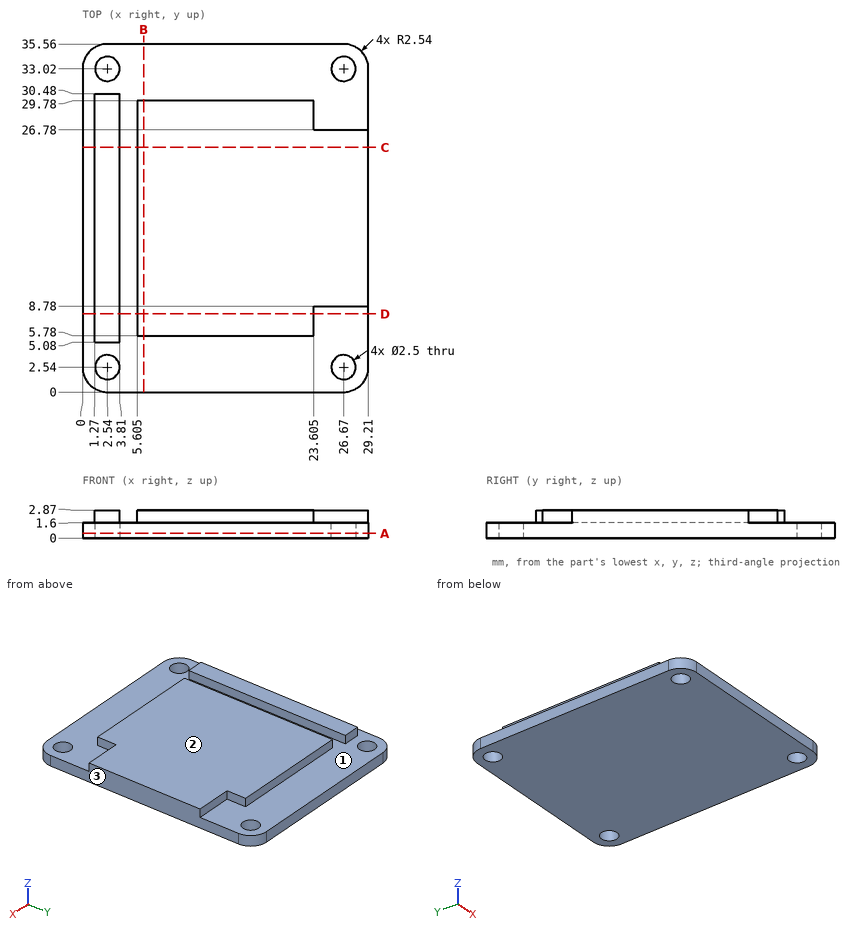
Geometry check sheet. Reference: drawing and pictorial views, mm from the part's lowest x, y, z. Give positions to 0.01 mm unless a question says otherwise; leave off trailing zeros. Write each loop counter-clockwise with the first axis right and the second up, starting at its lowest first coordinate (ties: lowest second). Pieces come first, ordered by that corner, then holes. Notation, with made-up numbers: M -22.75,50 L 18.25,50 A18 ccw 18.25,60 Z; hole C 60,65 d7. An arc over 180 degrees is marked long. Put each result on its own line as item: value. Start each with the question number.
1. Draft check along X on the marked faces 1, 2 and 3. Enter one of: +X half, -X half, draft (parallel to the pull), parting line (faces both ways), or undercut.
2. Section check D-D (y = 8). Record the cut outline in (x, z) (3 decimals).
3. Section check C-C (y = 25). Record the cut outline in (x, z) (3 decimals).
4. Section check A-A (z = 0.5). Record the cut outline in (x, y).
5. Section check B-B (x = 6.25). Record the cut outline in (y, z).
6. Go/stop test with flat-tipped pins: pin 1 Ø3 at (x, y) = (26.67, 33.02) entering from +Z; pin 2 Ø0.6 at (y, z) = (7.5, 2.5) entering from +X (3 decimals); pin 3 Ø0.6 at (y, z) = (20.5, 2) entering from -X. Record where each tip stops, or that it passes through.
7. Scan lines: line 1 along Y through (x, z) = (26.75, 1.2); line 2 along X through (y, z) = (33.02, 0.6); line 3 along X through (y, z) = (17, 2.75) (3 decimals). Record each from-to range of solid material in increasing order. Write a range as [from, to].
Answer list:
1. face 1: undercut
1. face 2: draft
1. face 3: +X half
2. outline: M 0,0 L 29.21,0 L 29.21,1.6 L 23.605,1.6 L 23.605,2.87 L 5.605,2.87 L 5.605,1.6 L 3.81,1.6 L 3.81,2.87 L 1.27,2.87 L 1.27,1.6 L 0,1.6 Z
3. outline: M 0,0 L 29.21,0 L 29.21,2.87 L 5.605,2.87 L 5.605,1.6 L 3.81,1.6 L 3.81,2.87 L 1.27,2.87 L 1.27,1.6 L 0,1.6 Z
4. outline: M 0,2.54 A2.54 ccw 2.54,0 L 26.67,0 A2.54 ccw 29.21,2.54 L 29.21,33.02 A2.54 ccw 26.67,35.56 L 2.54,35.56 A2.54 ccw 0,33.02 Z; hole C 2.54,2.54 d2.5; hole C 2.54,33.02 d2.5; hole C 26.67,2.54 d2.5; hole C 26.67,33.02 d2.5
5. outline: M 0,0 L 35.56,0 L 35.56,1.6 L 29.78,1.6 L 29.78,2.87 L 5.78,2.87 L 5.78,1.6 L 0,1.6 Z
6. pin 1: z = 1.6
6. pin 2: x = 23.605
6. pin 3: x = 1.27
7. line 1: [0, 1.29], [3.79, 31.77], [34.27, 35.56]
7. line 2: [0, 1.29], [3.79, 25.42], [27.92, 29.21]
7. line 3: [1.27, 3.81], [5.605, 29.21]
